Work out the finished part from the listing and answer in its coordinate system (mm). A direction names the side the tool comes from. Give positions to 0.01 mm unless a question says otherwise; leave off trailing zeros. Order: outer loops, then holes, each group sorted by start corner. A loop starts at its lowest first (then second) coordinate and runs counter-clockwise, first axis right, second up. Notation, with made-up numbers: (86.5, -23.5) -> (95.5, -23.5) arc R22 cw to (95.5, 15.5) -> close; hole circle Ø3 at (-8.75, 23). An arc over 180 degrees is marked (long way). Use a Markdown table: item, result. Add a question column.
```python
from build123d import *

# Parameters (mm, degrees)
SKETCH1_R           = 6.25
BOSS_EXTRUDE1_DEPTH = 38
SKETCH1_3_R         = 9.45
BOSS_EXTRUDE2_DEPTH = 16
FILLET1_R           = 2
CHAMFER1_SIZE       = 1
CUT_EXTRUDE4_DEPTH  = 6.35
CUT_EXTRUDE5_DEPTH  = 12.7
CUT_EXTRUDE6_REACH  = 6.45
SKETCH6_R           = 1.25


with BuildPart() as part:
    # Sketch1 → Boss-Extrude1 (new body)
    with BuildSketch(Plane(origin=(0, 0, 0), x_dir=(1, 0, 0), z_dir=(0, 1, 0))):
        Circle(SKETCH1_R)
    extrude(amount=BOSS_EXTRUDE1_DEPTH)

    # Sketch1_3 → Boss-Extrude2 (add)
    with BuildSketch(Plane(origin=(0, 0, 0), x_dir=(1, 0, 0), z_dir=(0, 1, 0))):
        Circle(SKETCH1_3_R)
    extrude(amount=BOSS_EXTRUDE2_DEPTH)

    # Fillet1
    fillet1_edges = [part.edges().sort_by_distance(p)[0] for p in [
        (-6.25, 16, 0),
    ]]
    fillet(fillet1_edges, radius=FILLET1_R)

    # Chamfer1
    chamfer1_edges = [part.edges().sort_by_distance(p)[0] for p in [
        (-6.25, 38, 0),
    ]]
    chamfer(chamfer1_edges, length=CHAMFER1_SIZE)

    # Sketch2 → Revolve1 (revolve)
    with BuildSketch(Plane(origin=(0, 0, 0), x_dir=(0, 0, -1), z_dir=(1, 0, 0))):
        with BuildLine():
            Line((0, 45), (0, 38))
            Line((0, 38), (7, 38))
            ThreePointArc((7, 38), (4.949747468, 42.949747468), (0, 45))
        make_face()
    revolve(axis=Axis((0, 47.571975937, 0), (0, -1, 0)))

    # Sketch3 → Cut-Extrude4 (cut)
    with BuildSketch(Plane(origin=(0, 38, 0), x_dir=(-1, 0, 0), z_dir=(0, -1, 0))):
        with BuildLine():
            Line((-3.75, 5), (3.75, 5))
            ThreePointArc((3.75, 5), (0, 6.25), (-3.75, 5))
        make_face()
    extrude(amount=CUT_EXTRUDE4_DEPTH, mode=Mode.SUBTRACT)

    # Sketch5 → Cut-Extrude5 (cut)
    with BuildSketch(Plane.XZ):
        with BuildLine():
            Line((4.153311931, -5), (-4.153311931, -5))
            ThreePointArc((-4.153311931, -5), (0, 6.5), (4.153311931, -5))
        make_face()
    extrude(amount=-CUT_EXTRUDE5_DEPTH, mode=Mode.SUBTRACT)

    # Sketch6 → Cut-Extrude6 (cut, up to next)
    with BuildSketch(Plane.XY.offset(-5), mode=Mode.PRIVATE) as cut_extrude6_sk1:
        with Locations((0, 6.35)):
            Circle(SKETCH6_R)
    cut_extrude6_tool1 = extrude(cut_extrude6_sk1.sketch, amount=-CUT_EXTRUDE6_REACH, mode=Mode.PRIVATE) & part.part
    add(cut_extrude6_tool1.solids().sort_by_distance((0, 6.35, -5))[0], mode=Mode.SUBTRACT)


solid = part.part
```
1) The part is cut by section D-D, the plane y = 6.35. Determine the outline of the cut face in (x, z).
2) The part is cut by section B-B, the plane z = 0. Determine the outline of the cut face in (x, y).
3) Flat-ended cylindrical pins translate along their axes: pin 1 (3 mm diameter, centred on y = 11.5, z = -3.5, fed in from +X); pin 2 (1.9 mm diameter, centred on x = -1, y = 35, fed in from -Z); pin 3 (10 mm diameter, centred on y = 31, z = -6, fed in from -X); pin 4 (4 mm diameter, centred on y = 10, z = -0.5, fed in from -X). Find the tip coordinate at first contact, or state that the pin passes through.
4) Determine the mould class of faces 1 (the flat face through (0, 35, -5)), 2 (the cylindrical face through (-0.223, 6.261, 6.496)), 3 (the cylindrical face through (-1.355, 27.367, 6.101)), 4 (the flat face through (0, 0, -6)) for opening direction Y: released by +Y, released by -Y, zero draft, split by the parting line, or undercut.
5) Straight lines are drawn through the part: line 1 (X direction, y = 3.5, z = 0); line 2 (Y direction, x = 0.25, z = -5.5); line 3 (Y direction, x = -5.25, z = 7.25). For each, find the intervals that lie inside material, in ascending order.
6) Which of the six approach directions +Z, -Z, +X, -X, +Y, -Y give full straight-line access (tool end or side, diameter ignored) to faces 5 (the flat face through (0.1, 31.65, -5.5)), 6 (the conical face through (-0.214, 37.84, 5.405)), 7 (the flat face through (0, 8, -5))?
7) The part is cut by section C-C, the plane y = 33. Determine the outline of the cut face in (x, z), then the cut area to 3 significant figures.
8) The part is cut by section A-A, the plane x = 0. Determine the outline of the cut face in (y, z), then the cut area to 3 significant figures.
A:
| question | item | result |
|---|---|---|
| 1 | outline | (-4.15, -5) arc R6.5 cw (long way) to (4.15, -5) -> (1.25, -5) -> (1.25, -9.37) arc R9.45 ccw (long way) to (-1.25, -9.37) -> (-1.25, -5) -> close |
| 2 | outline | (-9.45, 0) -> (-6.5, 0) -> (-6.5, 12.7) -> (6.5, 12.7) -> (6.5, 0) -> (9.45, 0) -> (9.45, 16) -> (8.25, 16) arc R2 cw to (6.25, 18) -> (6.25, 37) -> (5.25, 38) -> (7, 38) arc R7 ccw to (-7, 38) -> (-5.25, 38) -> (-6.25, 37) -> (-6.25, 18) arc R2 cw to (-8.25, 16) -> (-9.45, 16) -> close |
| 3 | pin 1 | x = 9.24 |
| 3 | pin 2 | z = -5 |
| 3 | pin 3 | x = -6.17 |
| 3 | pin 4 | x = -9.45 |
| 4 | face 1 | undercut |
| 4 | face 2 | zero draft |
| 4 | face 3 | undercut |
| 4 | face 4 | released by -Y |
| 5 | line 1 | -9.45 to -6.5, 6.5 to 9.45 |
| 5 | line 2 | 0 to 5.13, 7.57 to 31.65, 38 to 42.32 |
| 5 | line 3 | 0 to 16 |
| 6 | face 5 | -Z, +X, -X |
| 6 | face 6 | none |
| 6 | face 7 | -Y |
| 7 | outline | (-3.75, -5) -> (3.75, -5) arc R6.25 ccw (long way) to start |
| 7 | area | 116 mm^2 |
| 8 | outline | (0, -9.45) -> (5.1, -9.45) -> (5.1, -5) -> (0, -5) -> close; (0, 6.5) -> (12.7, 6.5) -> (12.7, -5) -> (7.6, -5) -> (7.6, -9.45) -> (16, -9.45) -> (16, -8.25) arc R2 cw to (18, -6.25) -> (31.65, -6.25) -> (31.65, -5) -> (38, -5) -> (38, -7) arc R7 ccw to (38, 7) -> (38, 5.25) -> (37, 6.25) -> (18, 6.25) arc R2 cw to (16, 8.25) -> (16, 9.45) -> (0, 9.45) -> close |
| 8 | area | 490 mm^2 |
